Read the model definition and answer for the solid it produces. Units are mm, in the model's axes. A direction names the side the tool comes from. Give positions to 0.01 mm unless a question says otherwise; leave off trailing zeros. Loops run counter-clockwise (first coordinate to the right, second up) from the corner with the lowest first, then second, coordinate; pieces in that order, holes last. Notation, with made-up numbers: (17, -9) -> (34, -9) arc R13 cw to (34, 16) -> close; hole circle Ø11 at (10.25, -29). An arc over 180 degrees is marked (long way). Return JSON: item names as keys, results as strings. Group by question number.
from build123d import *

# Parameters (mm, degrees)
BOSS_EXTRUDE1_DEPTH = 3.175


with BuildPart() as part:
    # Sketch1 → Boss-Extrude1 (new body)
    with BuildSketch(Plane.XY):
        with BuildLine():
            Line((-307.975, 0), (-304.8, 0))
            Line((-304.8, 0), (-304.8, 6.50875))
            ThreePointArc((-304.8, 6.50875), (-307.18125, 8.89), (-304.8, 11.27125))
            Line((-304.8, 11.27125), (-304.8, 17.78))
            Line((-304.8, 17.78), (-308.916961876, 17.162455719))
            ThreePointArc((-308.916961876, 17.162455719), (-312.786650336, 15.026442621), (-314.325, 10.882709878))
            Line((-314.325, 10.882709878), (-314.325, 6.35))
            ThreePointArc((-314.325, 6.35), (-312.465128061, 1.859871939), (-307.975, 0))
        make_face()
        with BuildLine():
            Line((-304.8, 0), (-288.925, 0))
            Line((-288.925, 0), (-288.925, 3.175))
            Line((-288.925, 3.175), (-276.225, 3.175))
            Line((-276.225, 3.175), (-276.225, 0))
            Line((-276.225, 0), (-266.7, 0))
            Line((-266.7, 0), (-266.7, 9.36625))
            ThreePointArc((-266.7, 9.36625), (-269.08125, 11.7475), (-266.7, 14.12875))
            Line((-266.7, 14.12875), (-266.7, 23.495))
            Line((-266.7, 23.495), (-304.8, 17.78))
            Line((-304.8, 17.78), (-304.8, 11.27125))
            ThreePointArc((-304.8, 11.27125), (-303.116201977, 10.573798023), (-302.41875, 8.89))
            ThreePointArc((-302.41875, 8.89), (-303.116201977, 7.206201977), (-304.8, 6.50875))
            Line((-304.8, 6.50875), (-304.8, 0))
        make_face()
        with BuildLine():
            Line((-266.7, 9.36625), (-266.7, 0))
            Line((-266.7, 0), (-263.525, 0))
            ThreePointArc((-263.525, 0), (-259.034871939, 1.859871939), (-257.175, 6.35))
            Line((-257.175, 6.35), (-257.175, 17.550209878))
            ThreePointArc((-257.175, 17.550209878), (-259.381267257, 22.361860214), (-264.466961876, 23.829955719))
            Line((-264.466961876, 23.829955719), (-266.7, 23.495))
            Line((-266.7, 23.495), (-266.7, 14.12875))
            ThreePointArc((-266.7, 14.12875), (-265.016201977, 13.431298023), (-264.31875, 11.7475))
            ThreePointArc((-264.31875, 11.7475), (-265.016201977, 10.063701977), (-266.7, 9.36625))
        make_face()
    extrude(amount=BOSS_EXTRUDE1_DEPTH)


solid = part.part
1. Section D-D on x = -282.5 is taken. Determine the outline of the cut face in (y, z) (3 decimals), then the cut area to 3 significant figures.
2. Section C-C on x = -260.5 is taken. Determine the outline of the cut face in (y, z) (3 decimals).
3. Determine the mould class of faces 3 (the flat face through (-299, 0, 2)), 4 (the flat face through (-276.225, 2, 2)), 5 (the cylindrical face through (-259.085, 1.811, 1.565)) for opening direction X: pulls with the +X half, pulls with the -X half, needs draft (parallel to the pull), parting line crosses it, or undercut.
4. Straight lines are drawn through the part: line 1 (X direction, y = 11, z = 0.4) (3 decimals); line 2 (X direction, y = 10.75, z = 1.8) (3 decimals); line 3 (X direction, y = 12.75, z = 1.65) (3 decimals). For each, find the intervals that lie inside material, in ascending order. Write a range as from..to.
5. Section B-B on x = -303 is taken. Determine the outline of the cut face in (y, z) (3 decimals), then the cut area to 3 significant figures.
6. Which of the six approach directions +Z, -Z, +X, -X, +Y, -Y give full straight-line access (tool end or side, diameter ignored) to faces 1 (the flat face through (-286, 12, 3.175)), 2 (the flat face through (-288.925, 2, 2))?
7. Section A-A on z = 2.05 is taken. State how many separate pieces and enclosed holes the cut face has, then the cut area to 3 significant figures.
Completed:
{
 "1": {"outline": "(3.175, 0) -> (21.125, 0) -> (21.125, 3.175) -> (3.175, 3.175) -> close", "area": "57.0 mm²"},
 "2": {"outline": "(0.767, 0) -> (23.133, 0) -> (23.133, 3.175) -> (0.767, 3.175) -> close"},
 "3": {"face 3": "needs draft", "face 4": "undercut", "face 5": "pulls with the +X half"},
 "4": {"line 1": "x = -314.324..-305.904, -303.696..-268.961, -264.439..-257.175", "line 2": "x = -314.325..-306.287, -303.313..-268.862, -264.538..-257.175", "line 3": "x = -314.044..-268.86, -264.54..-257.175"},
 "5": {"outline": "(0, 0) -> (7.331, 0) -> (7.331, 3.175) -> (0, 3.175) -> close; (10.449, 0) -> (18.05, 0) -> (18.05, 3.175) -> (10.449, 3.175) -> close", "area": "47.4 mm²"},
 "6": {"face 1": "+Z, +X, -X, +Y, -Y", "face 2": "+Z, -Z, -Y"},
 "7": {"separate pieces": "1", "enclosed holes": "2", "area": "1,070 mm²"}
}
